Autodesk Fusion 360 part; units mm, degrees
sketch "Sketch1" plane through (0, 0, 0) normal (0, 0, 1) x (1, 0, 0)
  line L0 (124.9201, 72.5503) -> (24.9201, 72.5503)
  line L1 (24.9201, 72.5503) -> (24.9201, 12.5503)
  line L2 (24.9201, 12.5503) -> (124.9201, 12.5503)
  line L3 (124.9201, 12.5503) -> (124.9201, 72.5503)
  line L4 (124.9201, 42.5503) -> (24.9201, 42.5503) construction
  line L5 (74.9201, 72.5503) -> (74.9201, 12.5503) construction
  line L6 (120.4201, 68.0503) -> (69.4201, 68.0503)
  line L7 (69.4201, 68.0503) -> (69.4201, 17.0503)
  line L8 (69.4201, 17.0503) -> (120.4201, 17.0503)
  line L9 (120.4201, 17.0503) -> (120.4201, 68.0503)
  line L10 (120.4201, 68.0503) -> (69.4201, 17.0503) construction
  line L11 (69.4201, 68.0503) -> (120.4201, 17.0503) construction
  line L12 (114.9201, 42.5503) -> (114.9201, 68.0503) construction
  line L13 (114.9201, 65.5503) -> (69.4201, 65.5503) construction
  circle A0 centre (114.9201, 65.5503) radius 2.25
  line L14 (69.4201, 22.5503) -> (120.4201, 22.5503) construction
  line L15 (94.9201, 68.0503) -> (94.9201, 17) construction
  line L16 (76.9201, 17.0503) -> (76.9201, 42.5503) construction
  circle A1 centre (76.9201, 22.5503) radius 2.25
  line L17 (118.3201, 67.5133) -> (114.9201, 69.4763)
  line L18 (114.9201, 69.4763) -> (111.5201, 67.5133)
  line L19 (111.5201, 67.5133) -> (111.5201, 63.5873)
  line L20 (111.5201, 63.5873) -> (114.9201, 61.6243)
  line L21 (114.9201, 61.6243) -> (118.3201, 63.5873)
  line L22 (118.3201, 63.5873) -> (118.3201, 67.5133)
  line L23 (80.3201, 24.5133) -> (76.9201, 26.4763)
  line L24 (76.9201, 26.4763) -> (73.5201, 24.5133)
  line L25 (73.5201, 24.5133) -> (73.5201, 20.5873)
  line L26 (73.5201, 20.5873) -> (76.9201, 18.6243)
  line L27 (76.9201, 18.6243) -> (80.3201, 20.5873)
  line L28 (80.3201, 20.5873) -> (80.3201, 24.5133)
  line L29 (67.4201, 68.0503) -> (26.9201, 68.0503)
  line L30 (26.9201, 68.0503) -> (26.9201, 48.5503)
  line L31 (26.9201, 48.5503) -> (67.4201, 48.5503)
  line L32 (67.4201, 48.5503) -> (67.4201, 68.0503)
  line L33 (28.1201, 49.7503) -> (66.2201, 49.7503)
  line L34 (66.2201, 49.7503) -> (66.2201, 66.8503)
  line L35 (66.2201, 66.8503) -> (28.1201, 66.8503)
  line L36 (28.1201, 66.8503) -> (28.1201, 49.7503)
  line L37 (67.4201, 68.0503) -> (72.4201, 68.0503)
  line L38 (72.4201, 68.0503) -> (72.4201, 70.0503)
  line L39 (72.4201, 70.0503) -> (67.4201, 70.0503)
  line L40 (67.4201, 70.0503) -> (67.4201, 68.0503)
  point P0 (94.9201, 42.5503)
  point P1 (114.9201, 65.5503)
  point P2 (76.9201, 22.5503)
  dimension "d1" = 100
  dimension "d2" = 60
  dimension "d3" = 51
  dimension "d4" = 51
  dimension "d5" = 45.5
  dimension "d6" = 23
  dimension "d7" = 4.5
  dimension "d8" = 20
  dimension "d10" = 18
  dimension "d11" = 4.5
  dimension "d18" = 3.4
  dimension "d19" = 3.4
  dimension "d22" = 19.5
  dimension "d23" = 2
  dimension "d24" = 2
  dimension "d25" = -1.2
  dimension "d26" = 5
  dimension "d27" = 2
extrude "Extrude1" add sketch "Sketch1" along normal blind 5 contours L0 L1 L2 L3 | L29 L30 L31 L32 | L6 L37 L38 L39 L40 | L6 L17 L18 | L33 L34 L35 L36
extrude "Extrude2" add sketch "Sketch1" along normal blind 15 contours L6 L7 L8 L9 L17 L18 L19 L20 L21 L22 L37 | L6 L17 L18 L19 L20 L21 L22 | L23 L24 L25 L26 L27 L28
extrude "Extrude3" add 1 faces at (103.4201, 68.0503, 8.3333) along direction (0, 1, 0) blind 4.5
extrude "Extrude4" cut sketch "Sketch1" along normal blind 3 contours L6 L17 L18 | L6 L17 L18 L19 L20 L21 L22 | L23 L24 L25 L26 L27 L28
extrude "Extrude5" add sketch "Sketch1" along normal blind 18 contours L6 L37 L38 L39 L40
sketch "Sketch2" plane through (0, 0, 0) normal (0, 0, 1) x (1, 0, 0)
extrude "Extrude6" cut 1 faces at (69.7535, 68.0503, 17) along direction (0, 1, 0) blind 1.8
extrude "Extrude7" add 1 faces at (69.7535, 70.0503, 17) along direction (0, 1, 0) blind 2.5
Source: CAD feature listing. Evaluate the final solid. Frame: model axes, mm. A direction names the side the tool comes from. Round coordinates to 2 decimals unless told otherwise and drop trailing zeros. Loops run counter-clockwise (first coordinate to the right, second up) from the corner with the lowest first, then second, coordinate; pieces in that order, holes last. Notation, with made-up numbers: (74, 11) -> (115, 11) arc R19 ccw to (115, 31) -> close; hole circle Ø2 at (52, 46). An arc over 180 degrees is marked (long way). Answer as a JSON object with one key per item and string values. Group by question number.
Q1. Mould query, pull axis X, two halves, no side actions, for faces 1 (the flat face through (124.92, 42, 2)), 2 (the flat face through (70, 71, 18)), 3 (the flat face through (116.596, 62.592, 1.479)). Classes: pulls with the +X half, pulls with the -X half, needs draft (parallel to the pull), parting line crosses it, or undercut.
Q2. Section query C-C (z = 6). Output: boundary loops of the cut face in (x, y), plus the area to 3 significant figures.
Q3. Section query D-D (y = 23.5). Output: boundary loops of the cut face in (x, z).
Q4. Access query for faces 4 (the flat face through (95, 17.05, 10)), 5 (the flat face through (72.42, 71, 16)), 6 (the cylindrical face through (78.13, 20.653, 8.916)), 7 (the flat face through (69.42, 43, 10)), 8 (the flat face through (75.244, 25.509, 1.479)). Directions: +Z, -Z, +X, -X, +Y, -Y. A direction counts if a zero-diameter tool reaches every point of the face in a straight line with its end or side. Return the directions, or none.
Q5. Contact query for flat-ended pins moving along their axis: P1, Ø8, axis at x = 69.5, y = 58.5, coming from the +Z side; P2, Ø5, axis at x = 114.92, y = 65.55, coming from the -Z side; P3, Ø8, axis at x = 88.5, z = 12.5, coming from the -Y side; P4, Ø2.5, axis at x = 76.92, y = 22.55, coming from the +Z side. Output: stop coordinate, or through.
Q6. Ray query, line 1 (X direction, y = 22.5, z = 5.75); line 2 (Z direction, x = 85.5, y = 36.5); line 3 (Y direction, x = 118.5, z = 9). Return the intervals inside material, ascending. Write a range as from..to.
Q7. Section query B-B (x = 88). Output: boundary loops of the cut face in (y, z), plus the area to 3 significant figures.
Q8. Section query A-A (y = 33). Output: boundary loops of the cut face in (x, z).
Completed:
{
 "1": {"face 1": "pulls with the +X half", "face 2": "needs draft", "face 3": "undercut"},
 "2": {"outline": "(67.42, 69.85) -> (69.42, 69.85) -> (69.42, 17.05) -> (120.42, 17.05) -> (120.42, 72.55) -> (67.42, 72.55) -> close; hole circle Ø4.5 at (76.92, 22.55); hole circle Ø4.5 at (114.92, 65.55)", "area": "2,800 mm²"},
 "3": {"outline": "(24.92, 0) -> (73.52, 0) -> (73.52, 3) -> (74.88, 3) -> (74.88, 15) -> (69.42, 15) -> (69.42, 5) -> (24.92, 5) -> close; (78.96, 3) -> (80.32, 3) -> (80.32, 0) -> (124.92, 0) -> (124.92, 5) -> (120.42, 5) -> (120.42, 15) -> (78.96, 15) -> close"},
 "4": {"face 4": "+Z, +X, -X, -Y", "face 5": "+Z, +X, +Y, -Y", "face 6": "+Z, -Z", "face 7": "+Z, -X, -Y", "face 8": "-Z"},
 "5": {"P1": "z = 15", "P2": "z = 3", "P3": "y = 17.05", "P4": "through"},
 "6": {"line 1": "69.42..74.67, 79.17..120.42", "line 2": "0..15", "line 3": "17.05..72.55"},
 "7": {"outline": "(12.55, 0) -> (72.55, 0) -> (72.55, 15) -> (17.05, 15) -> (17.05, 5) -> (12.55, 5) -> close", "area": "855 mm²"},
 "8": {"outline": "(24.92, 0) -> (124.92, 0) -> (124.92, 5) -> (120.42, 5) -> (120.42, 15) -> (69.42, 15) -> (69.42, 5) -> (24.92, 5) -> close"}
}
